Design review of the part shown in the three views and the two pictorial views. Dimensions are in mm from the part's minimum x, y and z. A direction names the side the tool comes from. Give positions to 0.01 mm unless a question says otherwise; leave off trailing zeros. Order: outer loops, then holes, each group sorted by start corner. A loop starts at its lowest first (then second) coordinate and runs counter-clockwise, first axis right, second up. Notation, with made-up numbers: (-32, -39) - (-3, -39) arc R10 ccw to (-3, -26) - close; hole circle Ø4 at (89.5, 59.25). An arc over 180 degrees is marked (long way). Put each result on its own line as item: value.
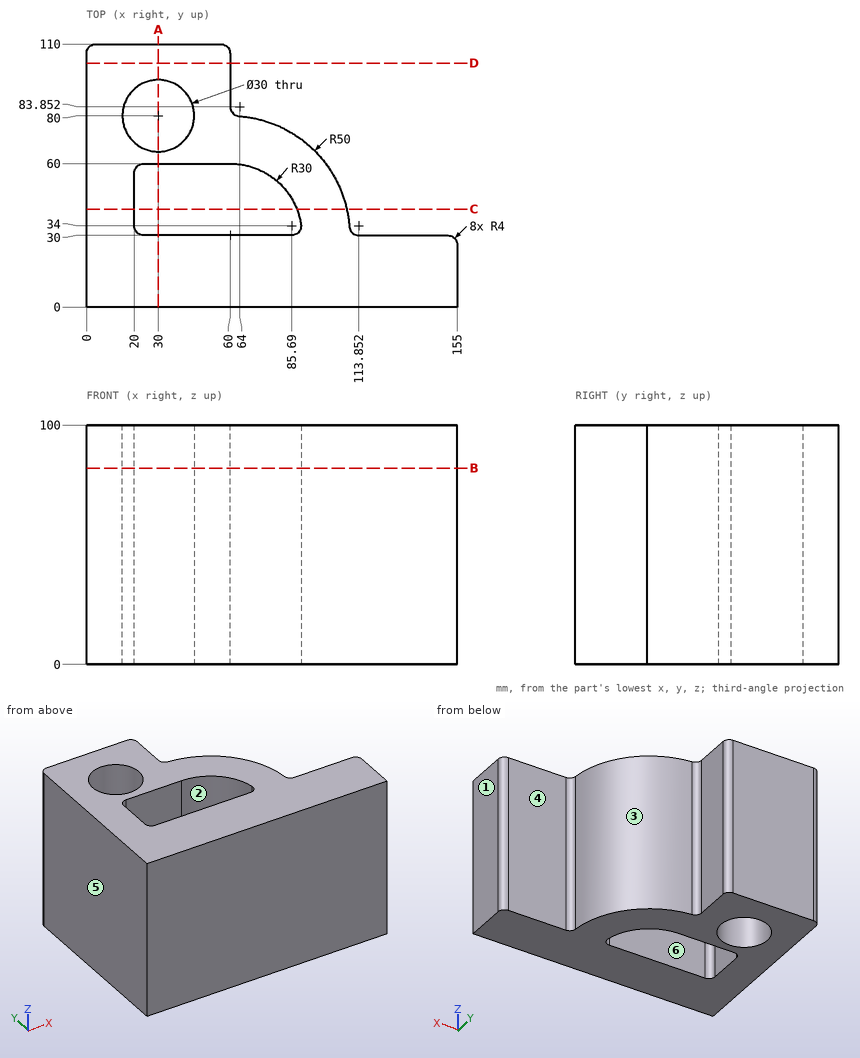
(1) Clearance check with flat-ended pins moving along their axes: pin 1 Ø11 at (x, z) = (134.5, 63.5) entering from +Y; pin 2 Ø2 at (x, z) = (87.5, 89) entering from +Y; pin 3 Ø24.5 at (y, z) = (97.5, 40) entering from +X. State where each tip first meets the part, or that it passes through.
The answers:
pin 1: y = 30
pin 2: y = 72.4
pin 3: x = 60
(2) The part is to be moulded in two halves that separate along Y. For the marked faces 1, 2 and 3, say which applies: pulls with the +Y half, pulls with the -Y half, needs draft (parallel to the pull), parting line crosses it, or undercut.
The answers:
face 1: needs draft
face 2: undercut
face 3: pulls with the +Y half
(3) Take a section at D-D, the plane y = 102. Write out the cut boundary in (x, z), then the cut area to 3 significant figures.
The answers:
outline: (0, 0) - (60, 0) - (60, 100) - (0, 100) - close
area: 6,000 mm^2
(4) Wall thickness on L1, parallel to Y at x = 30, z = 41; L2, parallel to Y at x = 47.5, z = 55; L3, parallel to Y at x = 135, z = 47: over which ranges is each line inside the solid? List them lowest first.
The answers:
L1: 0 to 30, 60 to 65, 95 to 110
L2: 0 to 30, 60 to 110
L3: 0 to 30
(5) Take a section at C-C, the plane y = 41. Write out the cut boundary in (x, z) (1 decimal).
The answers:
outline: (0, 0) - (20, 0) - (20, 100) - (0, 100) - close; (87.9, 0) - (108.8, 0) - (108.8, 100) - (87.9, 100) - close
(6) For the marked faces 4, 5 and 6, list the 3-axis set-ups (+Z, -Z, +X, -X, +Y, -Y) from which the entire face can be reached by the end or side of a thin tool; tool diameter is ignored.
The answers:
face 4: +Z, -Z, +X, +Y
face 5: +Z, -Z, -X, +Y, -Y
face 6: +Z, -Z
(7) Take a section at B-B, the plane z = 82. Write out the cut boundary in (x, y) (1 decimal), then the cut area to 3 significant figures.
The answers:
outline: (0, 0) - (155, 0) - (155, 26) arc R4 ccw to (151, 30) - (113.9, 30) arc R4 cw to (109.9, 33.7) arc R50 ccw to (63.7, 79.9) arc R4 cw to (60, 83.9) - (60, 106) arc R4 ccw to (56, 110) - (4, 110) arc R4 ccw to (0, 106) - close; hole circle Ø30 at (30, 80); hole (20, 34) arc R4 ccw to (24, 30) - (85.7, 30) arc R4 ccw to (89.6, 34.6) arc R30 ccw to (60, 60) - (24, 60) arc R4 ccw to (20, 56) - close
area: 8,810 mm^2
(8) Take a section at A-A, the plane x = 30. Write out the cut boundary in (y, z).
The answers:
outline: (0, 0) - (30, 0) - (30, 100) - (0, 100) - close; (60, 0) - (65, 0) - (65, 100) - (60, 100) - close; (95, 0) - (110, 0) - (110, 100) - (95, 100) - close
